Here's how the part is built. I have some questions about the finished solid (model axes, mm). A direction names the side the tool comes from. Give positions to 0.01 mm unless a question says otherwise; leave off trailing zeros. Loops run counter-clockwise (first coordinate to the right, second up) from the corner with the lowest first, then second, coordinate; pieces in that order, holes last.
Q1. I need wall thicknesses on probe 1 along X at (y, z) = (1, -1.25); probe 2 along X at (y, z) = (17.5, 1) (3 decimals); probe 3 along X at (y, z) = (-17.6, 0.3) (3 decimals). Which ranges of each line are inside material? Lowest first, please.
Q2. Suppose I cut it at D-D (x = -2.5). List the corners of the cut face in (y, z) for me, and give its area (3 significant figures).
Q3. I'm going to push a flat-ended pin straight in: P1, Ø2.5, axis at x = -5.345, y = 17.5, coming from the -Z side. Where does the tip first touch, or does it pass through?
Q4. Suppose I cut it at B-B (z = -2). List the corners of the cut face in (x, y) for me.
Q5. For faces 4 (the face through (-13.73, 0.28, 0.96)), 5 (the face through (12.75, 0, -7)), which set-ups out of +Z, -Z, +X, -X, +Y, -Y let a thin tool reach every point of the face, with its end or its side?
Q6. Suppose I cut it at A-A (y = 10). List the corners of the cut face in (x, z) for me (3 decimals), and give its area (3 significant figures).
Q7. Thinking about a two-plate mould opening in Y: for faces 1 (the face through (-1, 20, 0.2)), 2 (the face through (14.25, 0, -7)), 3 (the face through (13.51, 9.932, -8.454)), which applies, pulls with the +Y half, pulls with the -Y half, needs draft (parallel to the pull), parting line crosses it, or undercut?
Q8. Suppose I cut it at C-C (y = -10). List the corners of the cut face in (x, z) for me (3 decimals), and give its area (3 significant figures).
Autodesk Inventor part; units mm, degrees
ref_plane "YZ Plane" through (0, 0, 0) normal (1, 0, 0) x (0, 1, 0)
ref_plane "XZ Plane" through (0, 0, 0) normal (0, 1, 0) x (-1, 0, 0)
ref_plane "XY Plane" through (0, 0, 0) normal (0, 0, 1) x (1, 0, 0)
sketch "Sketch1" plane through (0, 0, 0) normal (0, 0, 1) x (1, 0, 0)
  line L0 (-14.25, -20) -> (14.25, -20)
  line L1 (14.25, -20) -> (14.25, 20)
  line L2 (14.25, 20) -> (-14.25, 20)
  line L3 (-14.25, 20) -> (-14.25, -20)
  line L4 (-14.25, -20) -> (14.25, 20) construction
  line L5 (14.25, -20) -> (-14.25, 20) construction
  point P0 (0, 0)
  dimension "d0" = 28.5
  dimension "d1" = 40
extrude "Plate1" add sketch "Sketch1" along normal blind 1.5
sketch "Sketch2" plane through (12.75, -20, 1.5) normal (1, 0, 0) x (0, 1, 0)
  line L0 (40, 0) -> (0, 0)
  line L1 (0, 0) -> (0, -15)
  line L2 (0, -15) -> (40, -15)
  line L3 (40, -15) -> (40, 0)
edge flange "Flange1" height 15 angle 90 thickness 1.5 bend radius 0.31 thickness toward (1, 0, 0) relief tear relief width 1.5 relief depth 0.75 corner gap 0.31 corner form 0 edges at (14.25, 0, 0) (-14.25, 0, 0) wall of the first edge with corners at (12.75, 20, 1.5) (12.75, -20, 1.5) (12.75, -20, -13.5) (12.75, 20, -13.5)
bend "Bend1"
corner "Corner1"
sketch "Sketch3" plane through (0, 0, 1.5) normal (0, 0, 1) x (1, 0, 0)
  ellipse E0 centre (-5.772, 17.882) end of major axis (-6.638, 18.748) minor radius 1 (-5.9956, 19) -> (-6.89, 18.1056) ccw
  line L0 (10.3556, 19) -> (-5.9956, 19)
  ellipse E1 centre (10.132, 17.882) end of major axis (10.998, 18.748) minor radius 1 (11.25, 18.1056) -> (10.3556, 19) ccw
  line L1 (11.25, -18.2056) -> (11.25, 18.1056)
  ellipse E2 centre (10.132, -17.982) end of major axis (10.998, -18.848) minor radius 1 (10.3556, -19.1) -> (11.25, -18.2056) ccw
  line L2 (-5.9956, -19.1) -> (10.3556, -19.1)
  ellipse E3 centre (-5.772, -17.982) end of major axis (-6.638, -18.848) minor radius 1 (-6.89, -18.2056) -> (-5.9956, -19.1) ccw
  line L3 (-6.89, 18.1056) -> (-6.89, -18.2056)
  circle A0 centre (9.705, -17.6) radius 0.7835
  circle A1 centre (-5.345, -17.6) radius 0.7835
  circle A2 centre (9.705, -2.5) radius 0.7835
  circle A3 centre (-5.345, -2.5) radius 0.7835
  circle A4 centre (9.705, 17.5) radius 0.7835
  circle A5 centre (-5.345, 17.5) radius 0.7835
  circle A6 centre (2.18, 10) radius 6.4
  point P0 (0, 0)
hole "Hole1" at (-5.345, -17.6, 1.5) at (9.705, -17.6, 1.5) at (9.705, -2.5, 1.5) at (-5.345, -2.5, 1.5) at (-5.345, 17.5, 1.5) at (9.705, 17.5, 1.5) direction (0, 0, -1) diameter 2.1 depth 1.5
sketch "Sketch4" plane through (0, 0, 1.5) normal (0, 0, 1) x (1, 0, 0)
  ellipse E0 centre (-5.772, 17.882) end of major axis (-6.638, 18.748) minor radius 1 (-5.9956, 19) -> (-6.89, 18.1056) ccw
  line L0 (10.3556, 19) -> (-5.9956, 19)
  ellipse E1 centre (10.132, 17.882) end of major axis (10.998, 18.748) minor radius 1 (11.25, 18.1056) -> (10.3556, 19) ccw
  line L1 (11.25, -18.2056) -> (11.25, 18.1056)
  ellipse E2 centre (10.132, -17.982) end of major axis (10.998, -18.848) minor radius 1 (10.3556, -19.1) -> (11.25, -18.2056) ccw
  line L2 (-5.9956, -19.1) -> (10.3556, -19.1)
  ellipse E3 centre (-5.772, -17.982) end of major axis (-6.638, -18.848) minor radius 1 (-6.89, -18.2056) -> (-5.9956, -19.1) ccw
  line L3 (-6.89, 18.1056) -> (-6.89, -18.2056)
  circle A0 centre (9.705, -17.6) radius 0.7835
  circle A1 centre (-5.345, -17.6) radius 0.7835
  circle A2 centre (9.705, -2.5) radius 0.7835
  circle A3 centre (-5.345, -2.5) radius 0.7835
  circle A4 centre (9.705, 17.5) radius 0.7835
  circle A5 centre (-5.345, 17.5) radius 0.7835
  circle A6 centre (2.18, 10) radius 6.4
  point P0 (0, 0)
extrude "Extrusion1" cut sketch "Sketch4" against normal blind 1.5 contours A6
fillet "Corner Round1" radius 1 4 edges at (13.5, 20, -13.5) (13.5, -20, -13.5) (-13.5, 20, -13.5) (-13.5, -20, -13.5)
sketch "Sketch5" plane through (-14.25, -20, -0.31) normal (-1, 0, 0) x (0, 0, 1)
  line L0 (-6.595, 40) -> (-6.595, 0)
  line L1 (-12.19, 40) -> (0, 40)
  line L2 (0, 0) -> (0, 40)
  circle A0 centre (-6.595, 30) radius 1.55
  circle A1 centre (-6.595, 10) radius 1.55
  line L3 (0, 0) -> (-12.19, 0)
  point P0 (0.31, 20)
  dimension "d23" = 40
  dimension "d24" = 6.595
  dimension "d25" = 3.1
  dimension "d26" = 3.1
  dimension "d27" = 10
  dimension "d28" = 10
hole "Hole2" at (-14.25, 10, -6.905) at (-14.25, -10, -6.905) direction (1, 0, 0) diameter 3.1 end through all
equation "\"d18\" = Thickness"
equation "\"d34\" = Thickness"
equation "\"d2\" = Thickness"
equation "\"d3\" = BendReliefWidth"
equation "\"d4\" = BendReliefDepth"
equation "\"d5\" = MinimumRemnant"
equation "\"d6\" = TransitionRadius"
equation "\"d9\" = BendRadius"
equation "\"d10\" = CornerReliefSize"
equation "\"d11\" = GapSize"
equation "\"d12\" = JacobiRadiusSize"
equation "\"BendReliefWidth\" = Thickness"
equation "\"BendReliefDepth\" = 0.5 * Thickness"
equation "\"CornerReliefSize\" = 4 * Thickness"
equation "\"MinimumRemnant\" = 2 * Thickness"
equation "\"TransitionRadius\" = BendRadius"
equation "\"JacobiRadiusSize\" = BendRadius"
equation "\"GapSize\" = Thickness"
properties part number "body_motor_L_frame" material "Aluminum 6061-AHC"
Solutions:
1. probe 1: x = -14.25 to -12.75, 12.75 to 14.25
1. probe 2: x = -13.689 to -6.395, -4.295 to 8.655, 10.755 to 13.689
1. probe 3: x = -14.144 to -6.395, -4.295 to 8.655, 10.755 to 14.144
2. outline: (-20, 0) - (5.63, 0) - (5.63, 1.5) - (-20, 1.5) - close; (14.37, 0) - (20, 0) - (20, 1.5) - (14.37, 1.5) - close
2. area: 46.9 mm2
3. P1: stops at z = 0
4. outline: (-14.25, -20) - (-12.75, -20) - (-12.75, 20) - (-14.25, 20) - close; (12.75, -20) - (14.25, -20) - (14.25, 20) - (12.75, 20) - close
5. face 4: +Z, -X, +Y, -Y
5. face 5: -Z, +Y, -Y
6. outline: (-14.25, -13.5) - (-12.75, -13.5) - (-12.75, -8.455) - (-14.25, -8.455) - close; (-14.25, -5.355) - (-12.75, -5.355) - (-12.75, -0.31) arc R0.31 cw to (-12.44, 0) - (-4.22, 0) - (-4.22, 1.5) - (-12.44, 1.5) arc R1.81 ccw to (-14.25, -0.31) - close; (8.58, 0) - (12.44, 0) arc R0.31 cw to (12.75, -0.31) - (12.75, -5.355) - (14.25, -5.355) - (14.25, -0.31) arc R1.81 ccw to (12.44, 1.5) - (8.58, 1.5) - close; (12.75, -13.5) - (14.25, -13.5) - (14.25, -8.455) - (12.75, -8.455) - close
6. area: 53.4 mm2
7. face 1: pulls with the +Y half
7. face 2: needs draft
7. face 3: undercut
8. outline: (-14.25, -13.5) - (-12.75, -13.5) - (-12.75, -8.455) - (-14.25, -8.455) - close; (-14.25, -5.355) - (-12.75, -5.355) - (-12.75, -0.31) arc R0.31 cw to (-12.44, 0) - (12.44, 0) arc R0.31 cw to (12.75, -0.31) - (12.75, -5.355) - (14.25, -5.355) - (14.25, -0.31) arc R1.81 ccw to (12.44, 1.5) - (-12.44, 1.5) arc R1.81 ccw to (-14.25, -0.31) - close; (12.75, -13.5) - (14.25, -13.5) - (14.25, -8.455) - (12.75, -8.455) - close
8. area: 72.6 mm2
